```python
from build123d import *

# Parameters (mm, degrees)
SKETCH1_W           = 80
SKETCH1_H           = 204
BOSS_EXTRUDE1_DEPTH = 3
SKETCH2_W           = 10
SKETCH2_H           = 3
BOSS_EXTRUDE2_DEPTH = 3
LPATTERN1_COUNT     = 4
LPATTERN1_PITCH     = 20
SKETCH3_W           = 10
SKETCH3_H           = 3
BOSS_EXTRUDE3_DEPTH = 3
LPATTERN2_COUNT     = 4
LPATTERN2_PITCH     = 20
SKETCH4_R           = 1.1
SKETCH4_R_2         = 1.5
SKETCH4_R_3         = 1.25
SKETCH4_W           = 10
SKETCH4_H           = 132.2
CUT_EXTRUDE1_DEPTH  = 4
SKETCH5_W           = 12
SKETCH5_H           = 3
SKETCH5_W_2         = 10
BOSS_EXTRUDE4_DEPTH = 3


with BuildPart() as part:
    # Sketch1 → Boss-Extrude1 (new body)
    with BuildSketch(Plane(origin=(0, 0, 0), x_dir=(1, 0, 0), z_dir=(0, 1, 0))):
        with Locations((40, 102)):
            Rectangle(SKETCH1_W, SKETCH1_H)
    extrude(amount=BOSS_EXTRUDE1_DEPTH)

    # Sketch2 → Boss-Extrude2 (add)
    with BuildSketch(Plane.XY):
        with Locations((5, 1.5)):
            Rectangle(SKETCH2_W, SKETCH2_H)
    boss_extrude2 = extrude(amount=BOSS_EXTRUDE2_DEPTH)

    # LPattern1: Boss-Extrude2 ×4
    with Locations(*[(i * LPATTERN1_PITCH, 0, 0) for i in range(1, LPATTERN1_COUNT)]):
        add(boss_extrude2)

    # Sketch3 → Boss-Extrude3 (add)
    with BuildSketch(Plane(origin=(0, 0, -204), x_dir=(-1, 0, 0), z_dir=(0, 0, -1))):
        with Locations((-5, 1.5)):
            Rectangle(SKETCH3_W, SKETCH3_H)
    boss_extrude3 = extrude(amount=BOSS_EXTRUDE3_DEPTH)

    # LPattern2: Boss-Extrude3 ×4
    with Locations(*[(i * LPATTERN2_PITCH, 0, 0) for i in range(1, LPATTERN2_COUNT)]):
        add(boss_extrude3)

    # Sketch4 → Cut-Extrude1 (cut, through all)
    with BuildSketch(Plane(origin=(0, 3, 0), x_dir=(1, 0, 0), z_dir=(0, 1, 0))):
        with Locations((20, 10)):
            Circle(SKETCH4_R)
        with Locations((67.5, 10)):
            Circle(SKETCH4_R)
        with Locations((20, 69.2)):
            Circle(SKETCH4_R)
        with Locations((67.5, 69.2)):
            Circle(SKETCH4_R)
        with Locations((20, 84.2)):
            Circle(SKETCH4_R_2)
        with Locations((69, 84.2)):
            Circle(SKETCH4_R_2)
        with Locations((69, 142.2)):
            Circle(SKETCH4_R_2)
        with Locations((20, 142.2)):
            Circle(SKETCH4_R_2)
        with Locations((48, 84.2)):
            Circle(SKETCH4_R_3)
        with Locations((48, 142.2)):
            Circle(SKETCH4_R_3)
        with Locations((9, 76.1)):
            Rectangle(SKETCH4_W, SKETCH4_H)
    extrude(amount=-CUT_EXTRUDE1_DEPTH, mode=Mode.SUBTRACT)

    # Sketch5 → Boss-Extrude4 (add)
    with BuildSketch(Plane.ZY):
        with Locations((-6, 1.5)):
            Rectangle(SKETCH5_W, SKETCH5_H)
        with Locations((-27, 1.5)):
            Rectangle(SKETCH5_W_2, SKETCH5_H)
        with Locations((-47, 1.5)):
            Rectangle(SKETCH5_W_2, SKETCH5_H)
        with Locations((-67, 1.5)):
            Rectangle(SKETCH5_W_2, SKETCH5_H)
        with Locations((-87, 1.5)):
            Rectangle(SKETCH5_W_2, SKETCH5_H)
        with Locations((-107, 1.5)):
            Rectangle(SKETCH5_W_2, SKETCH5_H)
        with Locations((-127, 1.5)):
            Rectangle(SKETCH5_W_2, SKETCH5_H)
        with Locations((-147, 1.5)):
            Rectangle(SKETCH5_W_2, SKETCH5_H)
        with Locations((-167, 1.5)):
            Rectangle(SKETCH5_W_2, SKETCH5_H)
        with Locations((-187, 1.5)):
            Rectangle(SKETCH5_W_2, SKETCH5_H)
    extrude(amount=BOSS_EXTRUDE4_DEPTH)


solid = part.part
```
For this review, take the finished solid that the model builds, in its own axes (mm). Coordinates: 2 decimals unless noted, no trailing zeros. Return JSON: item names as keys, results as strings. Group by question number.
(1) Consider section A-A, the plane y = 0.55. Count the separate pieces of the cut face and the enclosed holes in it, plus the area to 3 significant figures.
(2) For pin 1 Ø1.5 at (y, z) = (1.5, 2) entering from +X; pin 2 Ø0.9 at (y, z) = (2, -176.5) entering from -X; pin 3 Ø3.5 at (x, z) = (69, -84.2) entering from -Y; pin 4 Ø1.5 at (x, y) = (-2, 2) entering from -Z, all flat-tipped, find the tip position at first contact; note any pin that passes through.
(3) To check wall thickness, follow L1, parallel to Z at x = 69, y = 1.55; L2, parallel to X at y = 1.5, z = -69.2; L3, parallel to X at y = 0.85, z = -84.2. State the ranges of each line that lie inside material, in increasing order.
Results below:
{
 "1": {"separate pieces": "1", "enclosed holes": "11", "area": "15,500 mm2"},
 "2": {"pin 1": "stops at x = 70", "pin 2": "stops at x = 0", "pin 3": "stops at y = 0", "pin 4": "stops at z = -192"},
 "3": {"L1": "z = -207 to -143.7, -140.7 to -85.7, -82.7 to 3", "L2": "x = -3 to 4, 14 to 18.9, 21.1 to 66.4, 68.6 to 80", "L3": "x = -3 to 4, 14 to 18.5, 21.5 to 46.75, 49.25 to 67.5, 70.5 to 80"}
}
